Geometry check sheet. Reference: the model listing, model coordinates, mm. Face numbers are marked on the shaded views. Coordinates: 2 decimals unless noted, no trailing zeros. Loops run counter-clockwise (first coordinate to the right, second up) from the corner with the lowest first, then second, coordinate; pieces in that order, holes last. Notation, with made-up numbers: M 8.25,-25.75 L 15.25,-25.75 A30 ccw 15.25,6.25 Z; hole C 7,72.5 d8. An arc over 180 degrees is marked long. One line per question, with ' | ' between items. Start each with the question number.
from build123d import *

# Parameters (mm, degrees)
F1_DEPTH = 2
F2_R     = 1.79
F2_R_2   = 0.75
F3_DEPTH = 4
F5_DEPTH = 2


with BuildPart() as f1:
    # F0 (on Top) → F1 (new body)
    with BuildSketch(Plane.XY):
        with BuildLine():
            Line((10.7, 19.05), (-10.7, 19.05))
            ThreePointArc((-10.7, 19.05), (-12.114214, 18.464214), (-12.7, 17.05))
            Line((-12.7, 17.05), (-12.7, -17.05))
            ThreePointArc((-12.7, -17.05), (-12.114214, -18.464214), (-10.7, -19.05))
            Line((-10.7, -19.05), (10.7, -19.05))
            ThreePointArc((10.7, -19.05), (12.114214, -18.464214), (12.7, -17.05))
            Line((12.7, -17.05), (12.7, 17.05))
            ThreePointArc((12.7, 17.05), (12.114214, 18.464214), (10.7, 19.05))
        make_face()
    extrude(amount=F1_DEPTH)

    # F2 (on face) → F3 (join)
    with BuildSketch(Plane.XY.offset(2)):
        with Locations((-10.16, 16.51)):
            Circle(F2_R)
        with Locations((-10.16, 16.51)):
            Circle(F2_R_2, mode=Mode.SUBTRACT)
        with Locations((10.16, 16.51)):
            Circle(F2_R)
        with Locations((10.16, 16.51)):
            Circle(F2_R_2, mode=Mode.SUBTRACT)
        with Locations((10.16, -16.51)):
            Circle(F2_R)
        with Locations((10.16, -16.51)):
            Circle(F2_R_2, mode=Mode.SUBTRACT)
        with Locations((-10.16, -16.51)):
            Circle(F2_R)
        with Locations((-10.16, -16.51)):
            Circle(F2_R_2, mode=Mode.SUBTRACT)
    extrude(amount=F3_DEPTH)

    # F4 (on face) → F5 (cut)
    with BuildSketch(Plane.XY.offset(2)):
        with BuildLine():
            Line((6.168252, 13.253161), (-6.168252, 13.253161))
            ThreePointArc((-6.168252, 13.253161), (-7.582466, 12.667374), (-8.168252, 11.253161))
            Line((-8.168252, 11.253161), (-8.168252, -11.253161))
            ThreePointArc((-8.168252, -11.253161), (-7.582466, -12.667374), (-6.168252, -13.253161))
            Line((-6.168252, -13.253161), (6.168252, -13.253161))
            ThreePointArc((6.168252, -13.253161), (7.582466, -12.667374), (8.168252, -11.253161))
            Line((8.168252, -11.253161), (8.168252, 11.253161))
            ThreePointArc((8.168252, 11.253161), (7.582466, 12.667374), (6.168252, 13.253161))
        make_face()
    extrude(amount=-F5_DEPTH, mode=Mode.SUBTRACT)


solid = f1.part
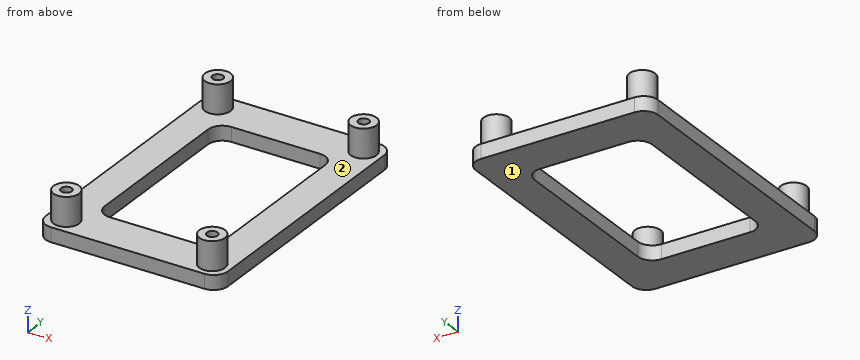
1. Thickness scan on line 1 (Y direction, x = 10.16, z = 4.05); line 2 (Y direction, x = -4.5, z = 1.05); line 3 (X direction, y = -17, z = 4.6). Record the ranges inside material, lowest first.
2. Sectioned sample at B-B (x = 1.5). Record the cut outline in (y, z).
3. Sectioned sample at A-A (z = 3.2). Record the cut outline in (x, y).
4. Sectioned sample at D-D (x = 10.16). Record the cut outline in (y, z).
5. Draft check along X on the marked faces 1 and 2. Enter one of: +X half, -X half, draft (parallel to the pull), parting line (faces both ways), or undercut.
6. Sectioned sample at C-C (y = 6). Record the cut outline in (x, z), and give its area (3 significant figures).
7. Depth check by flat-ended pin: pin 1 Ø0.9 at (x, y) = (10.16, -16.51) entering from -Z; pin 2 Ø6 at (x, y) = (-3.5, -4.5) entering from -Z; pin 3 Ø7.5 at (x, y) = (5.5, -7) entering from +Z. Enter the tip coordinate at first touch or a pass-through.
Result:
1) line 1: y = -18.3 to -17.26, -15.76 to -14.72, 14.72 to 15.76, 17.26 to 18.3 | line 2: y = -19.05 to -13.25, 13.25 to 19.05 | line 3: x = -11.88 to -10.73, -9.59 to -8.44, 8.44 to 9.59, 10.73 to 11.88
2) outline: M -19.05,0 L -13.25,0 L -13.25,2 L -19.05,2 Z; M 13.25,0 L 19.05,0 L 19.05,2 L 13.25,2 Z
3) outline: C -10.16,-16.51 d3.58; C -10.16,16.51 d3.58; C 10.16,-16.51 d3.58; C 10.16,16.51 d3.58; hole C -10.16,-16.51 d1.5; hole C -10.16,16.51 d1.5; hole C 10.16,-16.51 d1.5; hole C 10.16,16.51 d1.5
4) outline: M -19.05,0 L 19.05,0 L 19.05,2 L 18.3,2 L 18.3,6 L 17.26,6 L 17.26,2 L 15.76,2 L 15.76,6 L 14.72,6 L 14.72,2 L -14.72,2 L -14.72,6 L -15.76,6 L -15.76,2 L -17.26,2 L -17.26,6 L -18.3,6 L -18.3,2 L -19.05,2 Z
5) face 1: draft | face 2: undercut
6) outline: M -12.7,0 L -8.17,0 L -8.17,2 L -12.7,2 Z; M 8.17,0 L 12.7,0 L 12.7,2 L 8.17,2 Z | area: 18.1 mm2
7) pin 1: stops at z = 0 | pin 2: passes through | pin 3: stops at z = 2
